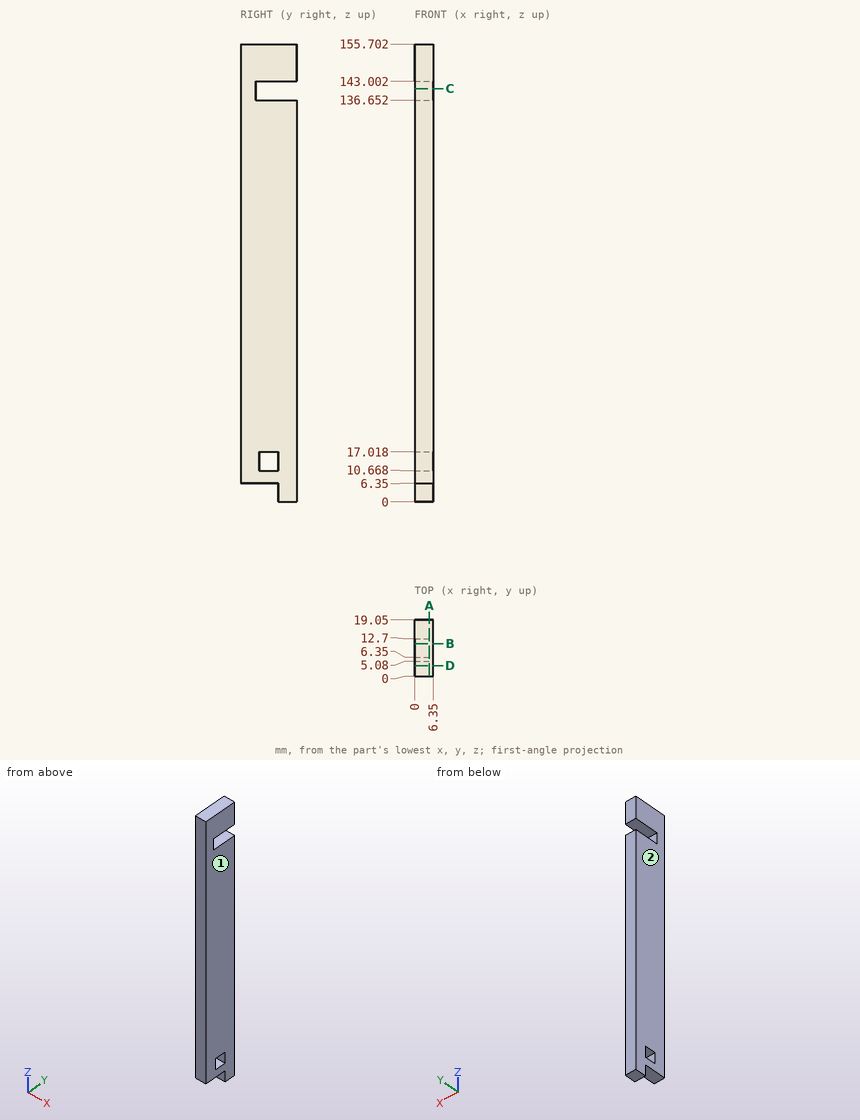
Verification items for this drawing (mm, ordinates from the low corner). Round coordinates to 2 decimals unless told otherwise and drop trailing zeros. Write each loop counter-clockwise with the first axis right and the second up, starting at its lowest first coordinate (ties: lowest second). Pieces come first, ordered by that corner, then holes. Notation, with made-up numbers: M -14,-3 L 2,-3 A15 cw 2,2 Z; hole C 49,82.25 d1. An arc over 180 degrees is marked long. Write item = value, one per line. Start each with the question number.
1. Release check for a two-part mould opening along X. For the marked faces 1 and 2 record: pulls with the +X half, pulls with the -X half, needs draft (parallel to the pull), parting line crosses it, or undercut.
2. Section check B-B, the plane y = 11. Record the cut outline in (x, z).
3. Scan lines: line 1 (Z direction, x = 1, y = 10.25); line 2 (Z direction, x = 0.5, y = 5.5); line 3 (Z direction, x = 6, y = 15). Record each from-to range of solid material in increasing order. Write a range as [from, to].
4. Section check A-A, the plane x = 5. Record the cut outline in (y, z), then the cut area to 3 significant figures.
5. Section check C-C, the plane z = 140.5. Record the cut outline in (x, y).
6. Gauge pin test, flat ends, axial feed: pin 1 (1.9 mm diameter, centred on x = 2, y = 9, fed in from -Z); pin 2 (1.9 mm diameter, centred on x = 3, z = 2, fed in from -Y). Record the tip position at first contact, or that the pin passes through.
7. Section check D-D, the plane y = 3.5. Record the cut outline in (x, z), then the cut area to 3 significant figures.
Results found:
q1.face_1 = pulls with the +X half
q1.face_2 = pulls with the -X half
q2.outline = M 0,6.35 L 6.35,6.35 L 6.35,10.67 L 0,10.67 Z; M 0,17.02 L 6.35,17.02 L 6.35,136.65 L 0,136.65 Z; M 0,143 L 6.35,143 L 6.35,155.7 L 0,155.7 Z
q3.line_1 = [6.35, 10.67], [17.02, 136.65], [143, 155.7]
q3.line_2 = [6.35, 136.65], [143, 155.7]
q3.line_3 = [0, 136.65], [143, 155.7]
q4.outline = M 0,6.35 L 12.7,6.35 L 12.7,0 L 19.05,0 L 19.05,136.65 L 5.08,136.65 L 5.08,143 L 19.05,143 L 19.05,155.7 L 0,155.7 Z; hole M 6.35,10.67 L 12.7,10.67 L 12.7,17.02 L 6.35,17.02 Z
q4.area = 2,760 mm^2
q5.outline = M 0,0 L 6.35,0 L 6.35,5.08 L 0,5.08 Z
q6.pin_1 = 6.35
q6.pin_2 = 12.7
q7.outline = M 0,6.35 L 6.35,6.35 L 6.35,155.7 L 0,155.7 Z
q7.area = 948 mm^2
